```python
from build123d import *

# Parameters (mm, degrees)
EXTRUDE_1_DEPTH = 20
FILLET_1_R      = 5


with BuildPart() as part:
    # 草圖1 → 填料-伸長1 (new body)
    with BuildSketch(Plane.XY):
        Polygon((30, 5), (15, 5), (5, 10), (5, 20), (0, 20), (0, 5), (0, 0), (5, 0), (30, 0), align=None)
    extrude(amount=EXTRUDE_1_DEPTH)

    # 圓角1
    fillet_1_edges = [part.edges().sort_by_distance(p)[0] for p in [
        (2.5, 20, 20),
        (2.5, 20, 0),
    ]]
    fillet(fillet_1_edges, radius=FILLET_1_R)


solid = part.part
```
CAD build for the part. Positions are in the model's coordinates, mm. A direction names the side the tool comes from. Give positions to 0.01 mm unless a question says otherwise; leave off trailing zeros. Order: outer loops, then holes, each group sorted by start corner. A loop starts at its lowest first (then second) coordinate and runs counter-clockwise, first axis right, second up. Notation, with made-up numbers: M -31.5,16.5 L -21.5,16.5 A13 cw -21.5,36.5 Z; hole C -21.5,-38 d2. An arc over 180 degrees is marked long. Put each result on its own line as item: value. Start each with the question number.
(1) Which spindle directions (+Z, -Z, +X, -X, +Y, -Y) get a long thin tool onto all of the face, cutting with end or side? Do faces 1 (the flat face through (5, 15, 10)), 2 (the flat face through (0, 10, 10)). Say none if no direction does.
(2) Saw through at B-B, the plane x = 2.5. Write the cut outline in (y, z), then the cut area to 3 significant figures.
(3) Flat gauge pins, fed straight in: pin 1 Ø6 at (x, y) = (25, 7) entering from -Z; pin 2 Ø6 at (x, y) = (18, 10.5) entering from +Z; pin 3 Ø8 at (y, z) = (17.5, 7) entering from +X; pin 4 Ø1.5 at (x, z) = (8.5, 7.5) entering from +Y (3 decimals). Where does each tip first touch, or does it go through?
(4) Saw through at D-D, the plane z = 17. Write the cut outline in (x, y).
(5) Saw through at C-C, the plane y = 13. Write the cut outline in (x, z), then the cut area to 3 significant figures.
(6) Saw through at A-A, the plane z = 7.75. Write the cut outline in (x, y).
(7) Drill centre lines: line 1 along X through (y, z) = (14.5, 1.5); line 2 along X through (y, z) = (7.5, 1.5). Where is each one in solid material? Low to high.
Check result:
1. face 1: +Z, -Z, +X, +Y
1. face 2: +Z, -Z, -X, +Y, -Y
2. outline: M 0,0 L 15,0 A5 ccw 20,5 L 20,15 A5 ccw 15,20 L 0,20 Z
2. area: 389 mm2
3. pin 1: stops at z = 0
3. pin 2: passes through
3. pin 3: stops at x = 5
3. pin 4: stops at y = 8.625
4. outline: M 0,0 L 30,0 L 30,5 L 15,5 L 5,10 L 5,19.58 L 0,19.58 Z
5. outline: M 0,0 L 5,0 L 5,20 L 0,20 Z
5. area: 100 mm2
6. outline: M 0,0 L 30,0 L 30,5 L 15,5 L 5,10 L 5,20 L 0,20 Z
7. line 1: x = 0 to 5
7. line 2: x = 0 to 10
